```python
from build123d import *


with BuildPart() as obj1:
    # Cone → Cone (revolve)
    with BuildSketch(Plane.XZ):
        Polygon((0, 0), (38, 0), (45, 50), (0, 50), align=None)
    revolve(axis=Axis((0, 0, 0), (0, 0, 1)))


with BuildPart() as obj2:
    # Cone001 → Cone001 (revolve)
    with BuildSketch(Plane.XZ):
        Polygon((0, 0), (41, 0), (48, 50), (0, 50), align=None)
    revolve(axis=Axis((0, 0, 0), (0, 0, 1)))

    # Cut: cut obj1
    add(obj1.part, mode=Mode.SUBTRACT)


solid = obj2.part
```
For this review, take the finished solid that the model builds, in its own axes (mm). Round coordinates to 2 decimals unless told otherwise and drop trailing zeros. Write each loop counter-clockwise with the first axis right and the second up, starting at its lowest first coordinate (ties: lowest second). Pieces come first, ordered by that corner, then holes. Notation, with made-up numbers: (-0.5, 8.5) -> (31.5, 8.5) arc R22 ccw to (31.5, 45.5) -> close; hole circle Ø2 at (76.5, 52). An arc over 180 degrees is marked (long way). Use one line per item in the form item = value.
1) Take a section at A-A, the plane x = 0. Write out the cut boundary in (y, z), and give its area (3 significant figures).
Found:
outline = (-48, 50) -> (-41, 0) -> (-38, 0) -> (-45, 50) -> close; (38, 0) -> (41, 0) -> (48, 50) -> (45, 50) -> close
area = 300 mm2
2) Take a section at D-D, the plane z = 25.5. Write out the cut boundary in (x, y).
Found:
outline = circle Ø89.14 at (0, 0); hole circle Ø83.14 at (0, 0)
3) Clearance check with flat-ended pins moving along their axes: pin 1 (1.5 mm diameter, centred on x = 13.5, z = 24.5, fed in from -Y); pin 2 (5 mm diameter, centred on y = 31.5, z = 37.5, fed in from +X); pin 3 (12 mm diameter, centred on y = -14, z = 42.5, fed in from +X). State where each tip first meets the part, or that it passes through.
Found:
pin_1 = -42.59
pin_2 = 36.08
pin_3 = 46.55
4) Take a section at C-C, the plane z = 14. Write out the cut boundary in (x, y).
Found:
outline = circle Ø85.92 at (0, 0); hole circle Ø79.92 at (0, 0)
5) To check wall thickness, follow L1, parallel to Y at x = 21.5, z = 46; L2, parallel to Y at x = 20, z = 8; L3, parallel to X at y = 23, z = 20. State the ranges of each line that lie inside material, in increasing order. Write a range as from..to.
Found:
L1 = -42.29..-38.89, 38.89..42.29
L2 = -37.07..-33.62, 33.62..37.07
L3 = -37.28..-33.7, 33.7..37.28
6) Mouldability with a two-part tool opening along X and no side actions: class faces 1 (the flat face through (14, 43, 50)), 2 (the conical face through (-8.84, -39.8, 19.79)), 3 (the conical face through (-9.49, -42.73, 19.79)) as +X half, -X half, draft (parallel to the pull), parting line (faces both ways), or undercut.
Found:
face_1 = draft
face_2 = undercut
face_3 = parting line
